```python
from build123d import *

# Parameters (mm, degrees)
F0_R     = 2.5
F1_DEPTH = 3.175


with BuildPart() as f1:
    # F0 (on Front) → F1 (new body, symmetric)
    with BuildSketch(Plane.XZ):
        with BuildLine():
            ThreePointArc((0, 47.625), (-6.35, 53.975), (-12.7, 47.625))
            Line((-12.7, 47.625), (-12.7, 0))
            Line((-12.7, 0), (0, 0))
            Line((0, 0), (0, 47.625))
        make_face()
        with Locations((-6.35, 47.625)):
            Circle(F0_R, mode=Mode.SUBTRACT)
        with BuildLine():
            Line((0, 0), (-12.7, 0))
            Line((-12.7, 0), (-12.7, -47.625))
            ThreePointArc((-12.7, -47.625), (-6.35, -53.975), (0, -47.625))
            Line((0, -47.625), (0, 0))
        make_face()
        with Locations((-6.35, -47.625)):
            Circle(F0_R, mode=Mode.SUBTRACT)
    extrude(amount=F1_DEPTH, both=True)


solid = f1.part
```
The listing builds one solid part. Answer for the finished solid, in the listing's coordinates (mm). Give positions to 0.01 mm unless a question says otherwise; leave off trailing zeros. Order: outer loops, then holes, each group sorted by start corner. A loop starts at its lowest first (then second) coordinate and runs counter-clockwise, first axis right, second up. Notation, with made-up numbers: M 38.5,8.5 L 46.5,8.5 A20 ccw 46.5,36.5 Z; hole C -16.75,-28 d4. An arc over 180 degrees is marked long. Put each result on its own line as item: value. Start each with the question number.
Item 1: Find the intervals of material crossed by line 1 along Z through (x, y) = (-6.35, 0) (3 decimals); line 2 along Z through (x, y) = (-5.5, 1.75); line 3 along Z through (x, y) = (-11.75, -1.5), in increasing order.
Item 2: The part is cut by section C-C, the plane x = -2. Determine the outline of the cut face in (y, z) (3 decimals), and give its area (3 significant figures).
Item 3: For a pull along X with two mould halves and no side action, classify faces 1 (the face through (-6.892, 0.044, -50.066)), 2 (the face through (-6.892, 0.044, 45.184)), 3 (the face through (-12.7, 0, 1)), 4 (the face through (-6, 3.175, 1)) as +X half, -X half, draft (parallel to the pull), parting line (faces both ways), or undercut.
Item 4: The part is cut by section B-B, the plane y = 0. Determine the outline of the cut face in (x, z) (3 decimals), and give its area (3 significant figures).
Item 5: Flat-ended cylindrical pins translate along their axes: P1, Ø1, axis at x = -5, y = 1.5, coming from the -Z side; P2, Ø1.5, axis at x = -5, y = 1.5, coming from the +Z side. Find the tip coordinate at first contact, or state that the pin passes through.
Item 6: The part is cut by section A-A, the plane x = -6.35. Determine the outline of the cut face in (y, z) (3 decimals), and give its area (3 significant figures).
Answer key:
1. line 1: z = -53.975 to -50.125, -45.125 to 45.125, 50.125 to 53.975
1. line 2: z = -53.92 to -49.98, -45.27 to 45.27, 49.98 to 53.92
1. line 3: z = -50.97 to 50.97
2. outline: M -3.175,-52.251 L 3.175,-52.251 L 3.175,52.251 L -3.175,52.251 Z
2. area: 664 mm²
3. face 1: undercut
3. face 2: undercut
3. face 3: -X half
3. face 4: draft
4. outline: M -12.7,-47.625 A6.35 ccw 0,-47.625 L 0,47.625 A6.35 ccw -12.7,47.625 Z; hole C -6.35,-47.625 d5; hole C -6.35,47.625 d5
4. area: 1,300 mm²
5. P1: stops at z = -53.92
5. P2: stops at z = 53.95
6. outline: M -3.175,-53.975 L 3.175,-53.975 L 3.175,-50.125 L -3.175,-50.125 Z; M -3.175,-45.125 L 3.175,-45.125 L 3.175,45.125 L -3.175,45.125 Z; M -3.175,50.125 L 3.175,50.125 L 3.175,53.975 L -3.175,53.975 Z
6. area: 622 mm²
